```python
from build123d import *

# Parameters (mm, degrees)
F0_R      = 17.5
F1_DEPTH  = 20
F2_R      = 7
F3_DEPTH  = 29
F4_R      = 4
F5_DEPTH  = 2
F7_DEPTH  = 3
F9_DEPTH  = 6
F10_W     = 4
F10_H     = 4
F11_DEPTH = 12.5


with BuildPart() as f1:
    # F0 (on Front) → F1 (new body, symmetric)
    with BuildSketch(Plane.XZ):
        Circle(F0_R)
    extrude(amount=F1_DEPTH, both=True)

    # F2 (on Top) → F3 (join)
    with BuildSketch(Plane.XY):
        Circle(F2_R)
    extrude(amount=F3_DEPTH)

    # F4 (on face) → F5 (join)
    with BuildSketch(Plane.XY.offset(29)):
        Circle(F4_R)
    extrude(amount=F5_DEPTH)

    # F6 (on face) → F7 (join)
    with BuildSketch(Plane.XY.offset(31)):
        with BuildLine():
            Line((-3, 2.6457513111), (-3, -2.6457513111))
            ThreePointArc((-3, -2.6457513111), (0, -4), (3, -2.6457513111))
            Line((3, -2.6457513111), (3, 2.6457513111))
            ThreePointArc((3, 2.6457513111), (0, 4), (-3, 2.6457513111))
        make_face()
    extrude(amount=F7_DEPTH)

    # F8 (on face) → F9 (join)
    with BuildSketch(Plane.XY.offset(34)):
        with BuildLine():
            ThreePointArc((-3, 0), (0, -3), (3, 0))
            ThreePointArc((3, 0), (0, 3), (-3, 0))
        make_face()
    extrude(amount=F9_DEPTH)

    # F10 (on Right) → F11 (join, symmetric)
    with BuildSketch(Plane.YZ):
        with Locations((0, 23)):
            Rectangle(F10_W, F10_H)
    extrude(amount=F11_DEPTH, both=True)


solid = f1.part
```
Input: part model. Units: mm. Frame: model coordinates. A direction names the side the tool comes from. Coordinates: 2 decimals unless noted, no trailing zeros. Loops run counter-clockwise (first coordinate to the right, second up) from the corner with the lowest first, then second, coordinate; pieces in that order, holes last. Notation, with made-up numbers: (32, 1.25) - (51, 1.25) arc R25 cw to (51, 33.25) - close; hole circle Ø3 at (86, 8). An arc over 180 degrees is marked (long way). Answer in a Markdown table with one row per item.
(1) Pin query (flat end, axial travel): P1, Ø2, axis at x = 10.5, y = -0.5, coming from the -Z side; P2, Ø12, axis at x = 14, y = -7.5, coming from the +Z side; P3, Ø1.2, axis at x = 9.5, z = 23, coming from the -Y side; P4, Ø4, axis at x = -2.5, y = -2.5, coming from the +Z side. Return the tip coordinate at first contact, or that it passes through.
Model answer:
| item | result |
|---|---|
| P1 | stops at z = -14.7 |
| P2 | stops at z = 25 |
| P3 | stops at y = -2 |
| P4 | stops at z = 40 |
(2) Cut plane C-C on y = 13.5. Output: boundary loops of the cut face in (x, z).
Model answer:
| item | result |
|---|---|
| outline | circle Ø35 at (0, 0) |
(3) Cut plane B-B on x = -8. Output: boundary loops of the cut face in (y, z), plus the area to 3 significant figures.
Model answer:
| item | result |
|---|---|
| outline | (-20, -15.56) - (20, -15.56) - (20, 15.56) - (-20, 15.56) - close; (-2, 21) - (2, 21) - (2, 25) - (-2, 25) - close |
| area | 1,260 mm² |
(4) Mould query, pull axis Z, two halves, no side actions, for faces 4 (the face through (-10, 0, 21)), 5 (the face through (0.2, 3.2, 34)), 6 (the face through (3, 0, 32)). Classes: pulls with the +Z half, pulls with the -Z half, needs draft (parallel to the pull), parting line crosses it, or undercut.
Model answer:
| item | result |
|---|---|
| face 4 | undercut |
| face 5 | pulls with the +Z half |
| face 6 | needs draft |
(5) Material intervals for L1, parallel to Z at x = -11.5, y = 0; L2, parallel to X at y = 9, z = 0.5; L3, parallel to Z at x = -3.5, y = -2.5, sorted ascending. Write a range as from..to.
Model answer:
| item | result |
|---|---|
| L1 | z = -13.19..13.19, 21..25 |
| L2 | x = -17.49..17.49 |
| L3 | z = -17.15..29 |
(6) Cut plane A-A on x = 0. Output: boundary loops of the cut face in (y, z).
Model answer:
| item | result |
|---|---|
| outline | (-20, -17.5) - (20, -17.5) - (20, 17.5) - (7, 17.5) - (7, 29) - (4, 29) - (4, 34) - (3, 34) - (3, 40) - (-3, 40) - (-3, 34) - (-4, 34) - (-4, 29) - (-7, 29) - (-7, 17.5) - (-20, 17.5) - close |
(7) Set-up query: faces 1 (the face through (10, 2, 23)), 2 (the face through (-10, -2, 23)), 3 (the face through (-3, 0, 32)). Return all of +Z, -Z, +X, -X, +Y, -Y with unobstructed straight access to the full face (end or side cutting, diameter ignored); none if empty.
Model answer:
| item | result |
|---|---|
| face 1 | +Z, +X, +Y |
| face 2 | +Z, -X, -Y |
| face 3 | +Z, -X, +Y, -Y |
(8) Cut plane D-D on z = 36. Output: boundary loops of the cut face in (x, y).
Model answer:
| item | result |
|---|---|
| outline | circle Ø6 at (0, 0) |
